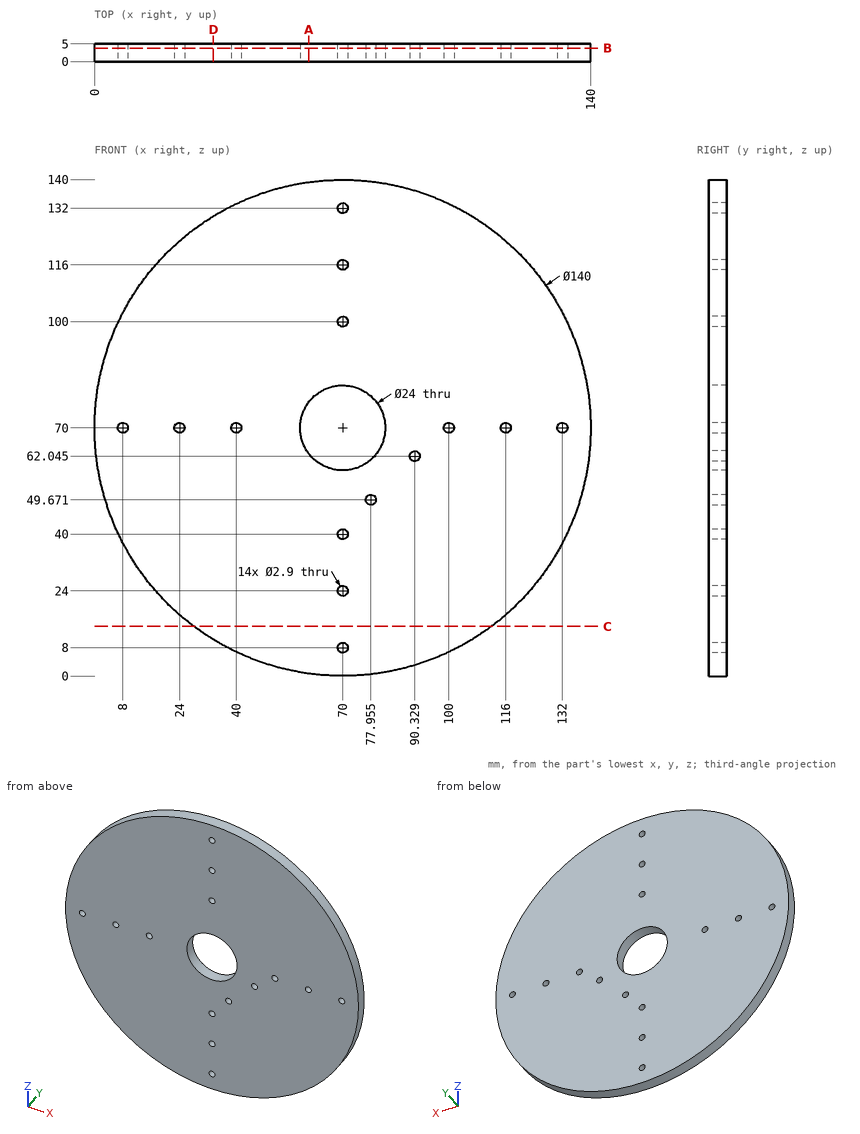
Part print with two shaded views. Sizes in mm from the minimum x, y, z corner. Coordinates: 2 decimals unless noted, no trailing zeros. Write each loop counter-clockwise with the first axis right and the second up, starting at its lowest first coordinate (ties: lowest second). Pieces come first, ordered by that corner, then holes. Notation, with made-up numbers: (73, 24) - (105, 24) arc R17 ccw to (105, 29) - close; hole circle Ø1 at (70, 54.25). An arc over 180 degrees is marked (long way). Use a Markdown table: item, result. Add a question column.
Item 1: Band-saw the part on A-A, the plane x = 60.5. Write the cut outline in (y, z).
Item 2: Drill centre lines: line 1 along X through (y, z) = (0.45, 76); line 2 along Z through (x, y) = (85, 1.85); line 3 along Z through (x, y) = (19, 0.4). Where is each one in solid material? Low to high.
Item 3: Band-saw the part on C-C, the plane z = 14. Write the cut outline in (x, y), and give its area (3 significant figures).
Item 4: Band-saw the part on D-D, the plane x = 33.5. Write the cut outline in (y, z), and give its area (3 significant figures).
Item 5: Band-saw the part on B-B, the plane y = 3.8. Give the number of separate pieces and of enclosed holes in the cut face, and give its area (3 significant figures).
A:
| question | item | result |
|---|---|---|
| 1 | outline | (0, 0.65) - (5, 0.65) - (5, 62.67) - (0, 62.67) - close; (0, 77.33) - (5, 77.33) - (5, 139.35) - (0, 139.35) - close |
| 2 | line 1 | x = 0.26 to 59.61, 80.39 to 139.74 |
| 2 | line 2 | z = 1.63 to 138.37 |
| 2 | line 3 | z = 22.05 to 117.95 |
| 3 | outline | (28, 0) - (112, 0) - (112, 5) - (28, 5) - close |
| 3 | area | 420 mm² |
| 4 | outline | (0, 10.27) - (5, 10.27) - (5, 129.73) - (0, 129.73) - close |
| 4 | area | 597 mm² |
| 5 | separate pieces | 1 |
| 5 | enclosed holes | 15 |
| 5 | area | 14,800 mm² |
